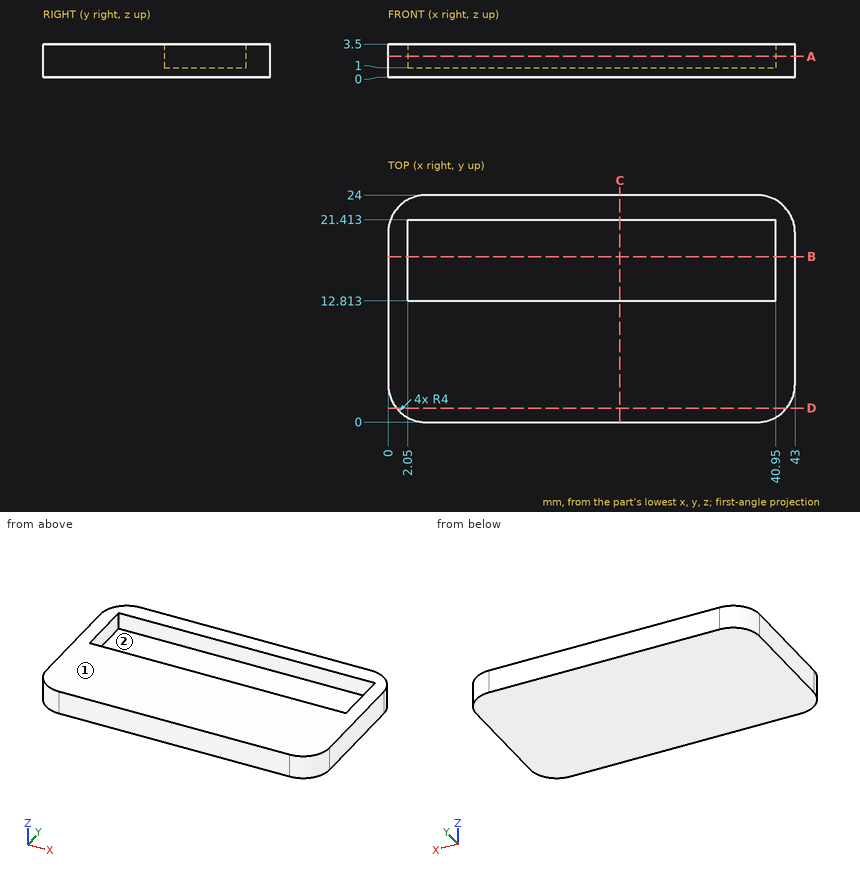
Study the drawing (mm; zero at the part's minimum x, y, z) and answer. A direction names the side the tool comes from. Give positions to 0.01 mm unless a question says otherwise; leave off trailing zeros. Write each loop counter-clockwise with the first axis right and the second up, starting at its lowest first coordinate (ties: lowest second). Pieces come first, ordered by that corner, then holes. Notation, with made-up numbers: (88.5, 77) -> (126.5, 77) arc R14 cw to (126.5, 93) -> close; hole circle Ø5 at (4.25, 15.5). An arc over 180 degrees is marked (long way). Write item = value, one per line. Start each with the question number.
1) The part is cut by section A-A, the plane z = 2.2. Determine the outline of the cut face in (x, y).
2) Straight lines are drawn through the part: line 1 along X through (y, z) = (16.25, 2.8); line 2 along Y through (x, z) = (34, 1.3); line 3 along Z through (x, y) = (14, 13.75). For each, find the intervals that lie inside material, in ascending order.
3) This flat-tipped pin is pushed along its axis until it touches: pin 1 (1.2 mm diameter, centred on x = 22.5, z = 2, fed in from -Y). Where does it stop, or does it pass through?
4) The part is cut by section C-C, the plane x = 24.5. Determine the outline of the cut face in (y, z).
5) The part is cut by section B-B, the plane y = 17.5. Determine the outline of the cut face in (x, z).
6) The part is cut by section D-D, the plane y = 1.5. Determine the outline of the cut face in (x, z), and give its area (3 significant figures).
7) Which of the six approach directions +Z, -Z, +X, -X, +Y, -Y give full straight-line access (tool end or side, diameter ignored) to the marked faces 1 and 2?
Solutions:
q1.outline = (0, 4) arc R4 ccw to (4, 0) -> (39, 0) arc R4 ccw to (43, 4) -> (43, 20) arc R4 ccw to (39, 24) -> (4, 24) arc R4 ccw to (0, 20) -> close; hole (2.05, 12.81) -> (40.95, 12.81) -> (40.95, 21.41) -> (2.05, 21.41) -> close
q2.line_1 = 0 to 2.05, 40.95 to 43
q2.line_2 = 0 to 12.81, 21.41 to 24
q2.line_3 = 0 to 1
q3.pin_1 = 0
q4.outline = (0, 0) -> (24, 0) -> (24, 3.5) -> (21.41, 3.5) -> (21.41, 1) -> (12.81, 1) -> (12.81, 3.5) -> (0, 3.5) -> close
q5.outline = (0, 0) -> (43, 0) -> (43, 3.5) -> (40.95, 3.5) -> (40.95, 1) -> (2.05, 1) -> (2.05, 3.5) -> (0, 3.5) -> close
q6.outline = (0.88, 0) -> (42.12, 0) -> (42.12, 3.5) -> (0.88, 3.5) -> close
q6.area = 144 mm²
q7.face_1 = +Z, +X, -X, +Y, -Y
q7.face_2 = +Z
